Design review of the part shown in the three views and the two pictorial views. Dimensions are in mm from the part's minimum x, y and z. A direction names the side the tool comes from. Coordinates: 2 decimals unless noted, no trailing zeros. Order: outer loops, then holes, each group sorted by start corner. A loop starts at its lowest first (then second) coordinate and runs counter-clockwise, first axis right, second up. Notation, with made-up numbers: (87, 13.5) -> (133, 13.5) arc R12 ccw to (133, 17.5) -> close; hole circle Ø2 at (62.5, 72). An arc over 180 degrees is marked (long way). Write item = value, one per line. Start each with the question number.
1) Consider section D-D on x = 3.5. Give the boundary of the cut face in (y, z).
2) Draft analysis for pull direction Z (two halves, no side actions). For the marked faces 3, 4 and 5, state which applies: +Z half, -Z half, draft (parallel to the pull), parting line (faces both ways), or undercut.
3) Consider section A-A on y = 12.5. Give the boundary of the cut face in (x, z).
4) Insertion check: pin 1 Ø6.5 at (y, z) = (4.27, 17.25) entering from +X; pin 2 Ø1.5 at (x, y) = (2, 16.5) entering from +Z; pin 3 Ø1.5 at (x, y) = (8, 14.5) entering from -Z. Each pin has a flat end and moves straight along its axis. Give the tip position at first contact, or say it passes through.
5) Consider section B-B on z = 12.5. Give the boundary of the cut face in (x, y), and give its area (4 significant figures).
6) Machinability: for the marked faces 1 and 2, which of the approach directions +Z, -Z, +X, -X, +Y, -Y give a long, thin tool a straight path to every point of the face, cutting with its end or side? Answer none if there is none.
7) Wall thickness on probe 1 along Y at (x, z) = (5, 17.25); probe 2 along Z at (x, y) = (5.75, 21.5) (1 decimal); probe 3 along X at (y, z) = (10.75, 24): over which ranges is each line inside the solid? List them lowest first. Write a range as [from, to].
8) Consider section C-C on y = 21.25. Give the boundary of the cut face in (x, z).
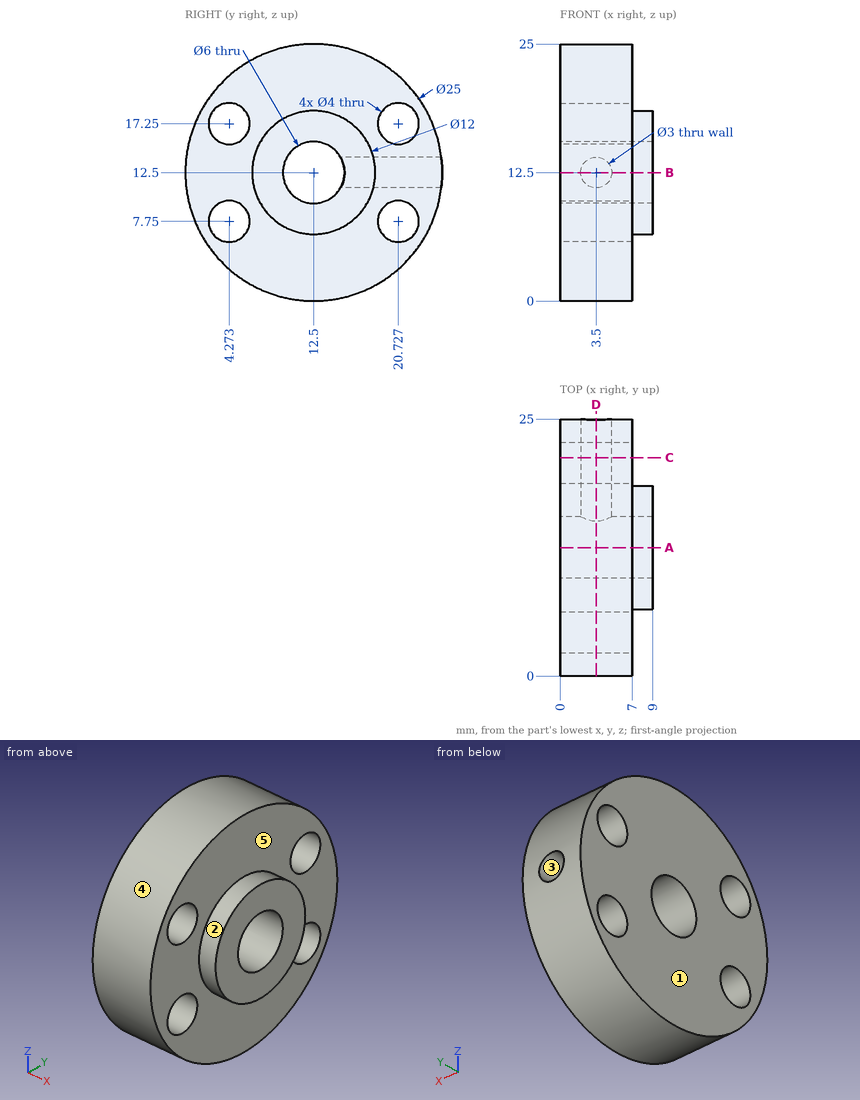
Answer sheet:
q1.outline = (15.1, 11) arc R3 cw (long way) to (15.1, 14) -> (24.91, 14) arc R12.5 ccw (long way) to (24.91, 11) -> close; hole circle Ø4 at (4.27, 7.75); hole circle Ø4 at (4.27, 17.25); hole circle Ø4 at (20.73, 7.75); hole circle Ø4 at (20.73, 17.25)
q2.face_3 = undercut
q2.face_4 = parting line
q2.face_5 = draft
q3.outline = (0, 0) -> (7, 0) -> (7, 6.5) -> (9, 6.5) -> (9, 9.5) -> (0, 9.5) -> close; (0, 15.5) -> (9, 15.5) -> (9, 18.5) -> (7, 18.5) -> (7, 25) -> (0, 25) -> close
q4.pin_1 = 7
q4.pin_2 = 24.57
q4.pin_3 = 6.63
q5.outline = (0, 0) -> (7, 0) -> (7, 6.5) -> (9, 6.5) -> (9, 9.5) -> (0, 9.5) -> close; (0, 15.5) -> (2, 15.5) -> (2, 25) -> (0, 25) -> close; (5, 15.5) -> (9, 15.5) -> (9, 18.5) -> (7, 18.5) -> (7, 25) -> (5, 25) -> close
q5.area = 116.5 mm2
q6.face_1 = +Z, -Z, -X, +Y, -Y
q6.face_2 = +X
q7.probe_1 = [0.94, 2.27], [6.27, 18.73], [22.73, 24.06]
q7.probe_2 = [3.8, 5.9], [9.6, 15.4], [19.1, 21.2]
q7.probe_3 = [0, 7]
q8.outline = (0, 3.57) -> (7, 3.57) -> (7, 5.82) -> (0, 5.82) -> close; (0, 9.68) -> (7, 9.68) -> (7, 15.32) -> (0, 15.32) -> close; (0, 19.18) -> (7, 19.18) -> (7, 21.43) -> (0, 21.43) -> close; hole circle Ø3 at (3.5, 12.5)
